from build123d import *

# Parameters (mm, degrees)
ESQUISSE1_R        = 2.1
ESQUISSE1_R_2      = 8
ESQUISSE1_W        = 5
ESQUISSE1_H        = 50
BOSS_EXTRU_1_DEPTH = 5


with BuildPart() as part:
    # Esquisse1 → Boss.-Extru.1 (new body)
    with BuildSketch(Plane.XY):
        Polygon((0, -3.53), (0, -35), (-5, -35), (-5, -85), (0, -85), (0, -100.4), (3.918484905, -100.4), (3.918484905, -97.5), (13.918484905, -97.5), (13.918484905, -107.5), (3.918484905, -107.5), (3.918484905, -104.6), (0, -104.6), (0, -120), (-5, -120), (-5, -170), (0, -170), (0, -185.4), (3.918484905, -185.4), (3.918484905, -182.5), (13.918484905, -182.5), (13.918484905, -192.5), (3.918484905, -192.5), (3.918484905, -189.6), (0, -189.6), (0, -205), (-5, -205), (-5, -255), (0, -255), (0, -286.47), (158.918484905, -286.47), (158.918484905, -255), (163.918484905, -255), (163.918484905, -205), (158.918484905, -205), (158.918484905, -189.6), (155, -189.6), (155, -192.5), (145, -192.5), (145, -182.5), (155, -182.5), (155, -185.4), (158.918484905, -185.4), (158.918484905, -170), (163.918484905, -170), (163.918484905, -120), (158.918484905, -120), (158.918484905, -104.6), (155, -104.6), (155, -107.5), (145, -107.5), (145, -97.5), (155, -97.5), (155, -100.4), (158.918484905, -100.4), (158.918484905, -85), (163.918484905, -85), (163.918484905, -35), (158.918484905, -35), (158.918484905, -3.53), align=None)
        with Locations((97.5, -145)):
            Circle(ESQUISSE1_R, mode=Mode.SUBTRACT)
        with Locations((120, -132)):
            Circle(ESQUISSE1_R_2, mode=Mode.SUBTRACT)
        with Locations(Location((120, -158, 0), (0, 0, 180))):
            Circle(ESQUISSE1_R_2, mode=Mode.SUBTRACT)
        with Locations((120, -217)):
            Circle(ESQUISSE1_R_2, mode=Mode.SUBTRACT)
        with Locations(Location((120, -243, 0), (0, 0, 180))):
            Circle(ESQUISSE1_R_2, mode=Mode.SUBTRACT)
        with Locations((97.5, -60)):
            Rectangle(ESQUISSE1_W, ESQUISSE1_H, mode=Mode.SUBTRACT)
        with Locations((97.5, -230)):
            Rectangle(ESQUISSE1_W, ESQUISSE1_H, mode=Mode.SUBTRACT)
    extrude(amount=BOSS_EXTRU_1_DEPTH)


solid = part.part
The model under review builds one solid part; all positions refer to its coordinate system, in mm. A direction names the side the tool comes from. Coordinates: 2 decimals unless noted, no trailing zeros. Write each loop counter-clockwise with the first axis right and the second up, starting at its lowest first coordinate (ties: lowest second). Pieces come first, ordered by that corner, then holes. Notation, with made-up numbers: M 82.5,85 L 116.5,85 A26 ccw 116.5,122 Z; hole C 21.5,18 d4. An arc over 180 degrees is marked long. Put each result on its own line as item: value.
1) For faces 1 (the flat face through (158.918, -271, 2)), 2 (the flat face through (9, -182.5, 2)), 3 (the flat face through (-2, -35, 2)), 4 (the flat face through (158.918, -112, 2)), list the 3-axis set-ups (+Z, -Z, +X, -X, +Y, -Y) from which the entire face can be reached by the end or side of a thin tool; tool diameter is ignored.
Computed:
face 1: +Z, -Z, +X, -Y
face 2: +Z, -Z
face 3: +Z, -Z, -X, +Y
face 4: +Z, -Z, +X
2) Draft analysis for pull direction X (two halves, no side actions). For faces 5 (the flat face through (97, -85, 2)), 6 (the flat face through (97, -35, 2)), 7 (the flat face through (-3, -170, 2)), 8 (the flat face through (0, -197, 2)), state which applies: released by +X, released by -X, zero draft, split by the parting line, or undercut.
Computed:
face 5: undercut
face 6: undercut
face 7: zero draft
face 8: released by -X
3) Clearance check with flat-ended pins moving along their axes: pin 1 Ø1.5 at (y, z) = (-183.5, 3.5) entering from -X; pin 2 Ø2.5 at (x, z) = (161.5, 1.5) entering from -Y. State where each tip first meets the part, or that it passes through.
Computed:
pin 1: stops at x = 0
pin 2: stops at y = -255
4) Add section C-C on z = 3.1. State how many separate pieces and enclosed holes the cut face has, then the cut area to 3 significant figures.
Computed:
separate pieces: 1
enclosed holes: 7
area: 44,700 mm2
5) Wall thickness on probe 1 along Y at (x, z) = (2, 3.4); probe 2 along Y at (x, z) = (120, 1.9); probe 3 along Y at (x, z) = (97.5, 2.15): over which ranges is each line inside the solid? List them lowest first. Write a range as [from, to].
Computed:
probe 1: y = [-286.47, -189.6], [-185.4, -104.6], [-100.4, -3.53]
probe 2: y = [-286.47, -251], [-235, -225], [-209, -166], [-150, -140], [-124, -3.53]
probe 3: y = [-286.47, -255], [-205, -147.1], [-142.9, -85], [-35, -3.53]
6) Add section B-B on y = -243. Give the boundary of the cut face in (x, z), then the cut area to 3 significant figures.
Computed:
outline: M -5,0 L 95,0 L 95,5 L -5,5 Z; M 100,0 L 112,0 L 112,5 L 100,5 Z; M 128,0 L 163.92,0 L 163.92,5 L 128,5 Z
area: 740 mm2
7) Add section A-A on y = -41. Give the boundary of the cut face in (x, z).
Computed:
outline: M -5,0 L 95,0 L 95,5 L -5,5 Z; M 100,0 L 163.92,0 L 163.92,5 L 100,5 Z
8) Add section D-D on y = -132. Give the boundary of the cut face in (x, z), then the cut area to 3 significant figures.
Computed:
outline: M -5,0 L 112,0 L 112,5 L -5,5 Z; M 128,0 L 163.92,0 L 163.92,5 L 128,5 Z
area: 765 mm2
